from build123d import *

# Parameters (mm, degrees)
SKETCH1_W           = 1118.25
SKETCH1_H           = 944.035
BOSS_EXTRUDE1_DEPTH = 15.875
BOSS_EXTRUDE3_REACH = 961.91
SKETCH3_W           = 15.875
SKETCH3_H           = 15.875


with BuildPart() as part:
    # Sketch1 → Boss-Extrude1 (new body)
    with BuildSketch(Plane(origin=(0, 0, 0), x_dir=(0, 0, -1), z_dir=(1, 0, 0))):
        Polygon((-575, -487.8925), (-575, 487.8925), (575, 487.8925), (575, -487.8925), (559.125, -487.8925), (-559.125, -487.8925), align=None)
        Rectangle(SKETCH1_W, SKETCH1_H, mode=Mode.SUBTRACT)
    extrude(amount=BOSS_EXTRUDE1_DEPTH)

    # Sketch3 → Boss-Extrude3 (add, up to next)
    with BuildSketch(Plane(origin=(0, -472.0175, 0), x_dir=(1, 0, 0), z_dir=(0, 1, 0)), mode=Mode.PRIVATE) as boss_extrude3_sk1:
        with Locations((7.9375, 16.375)):
            Rectangle(SKETCH3_W, SKETCH3_H)
    boss_extrude3_tool1 = extrude(boss_extrude3_sk1.sketch, amount=BOSS_EXTRUDE3_REACH, mode=Mode.PRIVATE) - part.part
    add(boss_extrude3_tool1.solids().sort_by_distance((7.9375, -472.0175, -16.375))[0])


solid = part.part
Source: CAD feature listing. Evaluate the final solid. Frame: model axes, mm. Coordinates: 2 decimals unless noted, no trailing zeros. Loops run counter-clockwise (first coordinate to the right, second up) from the corner with the lowest first, then second, coordinate; pieces in that order, holes last. Notation, with made-up numbers: M -18,-26.5 L 35,-26.5 A33 ccw 35,1.5 Z; hole C -28,5.5 d2. An arc over 180 degrees is marked long. Answer in a Markdown table with one row per item.
Q1. Section B-B on y = 287. Return the cut outline in (x, z) (1 decimal), plus the area to 3 significant figures.
Answers below:
| item | result |
|---|---|
| outline | M 0,-575 L 15.9,-575 L 15.9,-559.1 L 0,-559.1 Z; M 0,-24.3 L 15.9,-24.3 L 15.9,-8.4 L 0,-8.4 Z; M 0,559.1 L 15.9,559.1 L 15.9,575 L 0,575 Z |
| area | 756 mm^2 |
Q2. Section C-C on x = 10.5. Return the cut outline in (y, z) (1 decimal), plus the area to 3 significant figures.
Answers below:
| item | result |
|---|---|
| outline | M -487.9,-575 L 487.9,-575 L 487.9,575 L -487.9,575 Z; hole M -472,-559.1 L 472,-559.1 L 472,-24.3 L -472,-24.3 Z; hole M -472,-8.4 L 472,-8.4 L 472,559.1 L -472,559.1 Z |
| area | 81,500 mm^2 |
Q3. Section A-A on z = 350.5. Return the cut outline in (x, y) (1 decimal).
Answers below:
| item | result |
|---|---|
| outline | M 0,-487.9 L 15.9,-487.9 L 15.9,-472 L 0,-472 Z; M 0,472 L 15.9,472 L 15.9,487.9 L 0,487.9 Z |
Q4. First-contact query: pin 1 (1.5 mm diameter, centred on y = 230.5, z = -8.5, fed in from -X). Flat tip, straight axial feed; report the tip coordinate or a pass-through.
Answers below:
| item | result |
|---|---|
| pin 1 | stops at x = 0 |
Q5. Ray query, probe 1 along Z at (x, y) = (3.5, 307) (1 decimal); probe 2 along Y at (x, z) = (7, 468.5). Return the intervals inside material, ascending. Write a range as from..to.
Answers below:
| item | result |
|---|---|
| probe 1 | z = -575..-559.1, -24.3..-8.4, 559.1..575 |
| probe 2 | y = -487.89..-472.02, 472.02..487.89 |
